from build123d import *

# Parameters (mm, degrees)
F0_R     = 37
F0_R_2   = 10.95
F1_DEPTH = 7


# Not quite as in the source:
# - a fillet or chamfer that OpenCascade refuses, or shapes differently, is made with other operations: its cross-section is extruded or revolved along the edge and cut away or added


with BuildPart() as f1:
    # F0 (on Top) → F1 (new body)
    with BuildSketch(Plane.XY):
        Circle(F0_R)
        Polygon((-15.9939083851, -27.3076168841), (-24.9167489583, -24.9167489583), (-27.3076168841, -15.9939083851), (-20.7756442366, -9.4619357376), (-11.8528036634, -11.8528036634), (-9.4619357376, -20.7756442366), align=None, mode=Mode.SUBTRACT)
        Polygon((8, -30.6188021535), (0, -35.237604307), (-8, -30.6188021535), (-8, -21.3811978465), (0, -16.762395693), (8, -21.3811978465), align=None, mode=Mode.SUBTRACT)
        Polygon((27.3076168841, -15.9939083851), (24.9167489583, -24.9167489583), (15.9939083851, -27.3076168841), (9.4619357376, -20.7756442366), (11.8528036634, -11.8528036634), (20.7756442366, -9.4619357376), align=None, mode=Mode.SUBTRACT)
        Polygon((-30.6188021535, -8), (-35.237604307, 0), (-30.6188021535, 8), (-21.3811978465, 8), (-16.762395693, 0), (-21.3811978465, -8), align=None, mode=Mode.SUBTRACT)
        Polygon((-27.3076168841, 15.9939083851), (-24.9167489583, 24.9167489583), (-15.9939083851, 27.3076168841), (-9.4619357376, 20.7756442366), (-11.8528036634, 11.8528036634), (-20.7756442366, 9.4619357376), align=None, mode=Mode.SUBTRACT)
        Circle(F0_R_2, mode=Mode.SUBTRACT)
        Polygon((15.9939083851, 27.3076168841), (24.9167489583, 24.9167489583), (27.3076168841, 15.9939083851), (20.7756442366, 9.4619357376), (11.8528036634, 11.8528036634), (9.4619357376, 20.7756442366), align=None, mode=Mode.SUBTRACT)
        Polygon((30.6188021535, 8), (35.237604307, 0), (30.6188021535, -8), (21.3811978465, -8), (16.762395693, 0), (21.3811978465, 8), align=None, mode=Mode.SUBTRACT)
        Polygon((0, 35.237604307), (8, 30.6188021535), (8, 21.3811978465), (0, 16.762395693), (-8, 21.3811978465), (-8, 30.6188021535), align=None, mode=Mode.SUBTRACT)
    extrude(amount=F1_DEPTH)

    # F2: fillet of radius 2 on 2 edges, made by hand

    # F2_s1 → F2_t2 (revolve, cut)
    with BuildSketch(Plane.XZ):
        with BuildLine():
            ThreePointArc((37, 5), (36.4142135624, 6.4142135624), (35, 7))
            Line((35, 7), (37, 7))
            Line((37, 7), (37, 5))
        make_face()
    revolve(axis=Axis((0, 0, 7), (0, 0, 1)), mode=Mode.SUBTRACT)

    # F2_s3 → F2_t4 (revolve, cut)
    with BuildSketch(Plane.XZ):
        with BuildLine():
            ThreePointArc((37, 2), (36.4142135624, 0.5857864376), (35, 0))
            Line((35, 0), (37, 0))
            Line((37, 0), (37, 2))
        make_face()
    revolve(axis=Axis((0, 0, 0), (0, 0, 1)), mode=Mode.SUBTRACT)


solid = f1.part
Design review of the part built by this model. Coordinates are the model's own, in mm. Coordinates: 2 decimals unless noted, no trailing zeros. Write each question's results on one line, items separated by ' | '. Start each with the question number.
(1) Clearance check with flat-ended pins moving along their axes: P1, Ø2, axis at y = -26, z = 4.5, coming from the +X side; P2, Ø2, axis at y = -23.5, z = 4, coming from the -X side; P3, Ø3.5, axis at x = 27, z = 3, coming from the -Y side; P4, Ø17.5, axis at x = 0, y = 0, coming from the -Z side. State where each tip first meets the part, or that it passes through.
(2) For line 1 along Y through (x, z) = (0, 3); line 2 along Y through (x, z) = (17, 5); line 3 along X through (y, z) = (23, 6), list the stretches that pass through material, from the lowest coordinate up. Write a range as from..to.
(3) Take a section at A-A on z = 4. Give the number of separate pieces and of enclosed holes in the cut face, and give its area (3 significant figures).
(4) The part is to be moulded in two halves that separate along X. For faces 1 (the face through (24.087, 12.774, 3.451)), 2 (the face through (-8.02, -36.12, 3.48)), 3 (the face through (8, 8, 0)), say which applies: pulls with the +X half, pulls with the -X half, needs draft (parallel to the pull), parting line crosses it, or undercut.
Results found:
1) P1: stops at x = 27.28 | P2: stops at x = -29.37 | P3: stops at y = -27.05 | P4: passes through
2) line 1: y = -37..-35.24, -16.76..-10.95, 10.95..16.76, 35.24..37 | line 2: y = -32.86..-27.04, -10.47..-0.41, 0.41..10.47, 27.04..32.86 | line 3: x = -28.64..-25.43, -11.69..-8, 8..11.69, 25.43..28.64
3) separate pieces: 1 | enclosed holes: 9 | area: 2,150 mm2
4) face 1: undercut | face 2: parting line crosses it | face 3: needs draft
